from build123d import *

# Parameters (mm, degrees)
SKETCH1_W               = 120
SKETCH1_H               = 110
SKETCH1_R               = 2.15
SKETCH1_R_2             = 1.65
BOSS_EXTRUDE1_DEPTH     = 3
SKETCH2_R               = 3
SKETCH2_R_2             = 1.65
BOSS_EXTRUDE2_DEPTH     = 6.6
CHAMFER5_SIZE           = 1.6
CHAMFER5_SIZE2          = 2.771281292
CUT_EXTRUDE1_DEPTH      = 4
SKETCH4_R               = 7
SKETCH4_R_2             = 2.15
BOSS_EXTRUDE3_DEPTH     = 9
CUT_EXTRUDE2_DEPTH      = 5
CHAMFER2_SIZE           = 0.4
SKETCH6_W               = 9
SKETCH6_H               = 16
BOSS_EXTRUDE4_DEPTH     = 6
CUT_EXTRUDE3_DEPTH      = 126.87295182
CUT_EXTRUDE3_DEPTH_BACK = 126.87295182
SKETCH8_W               = 13
SKETCH8_H               = 10
SKETCH8_R               = 2.15
BOSS_EXTRUDE5_DEPTH     = 10
CUT_EXTRUDE5_DEPTH      = 5
CHAMFER9_SIZE           = 3


with BuildPart() as part:
    # Sketch1 → Boss-Extrude1 (new body)
    with BuildSketch(Plane.XY):
        Rectangle(SKETCH1_W, SKETCH1_H)
        with Locations((-39, 39)):
            Circle(SKETCH1_R, mode=Mode.SUBTRACT)
        with Locations((39, 39)):
            Circle(SKETCH1_R, mode=Mode.SUBTRACT)
        with Locations((39, -39)):
            Circle(SKETCH1_R, mode=Mode.SUBTRACT)
        with Locations((-39, -39)):
            Circle(SKETCH1_R, mode=Mode.SUBTRACT)
        with Locations((33.07, 14.94)):
            Circle(SKETCH1_R_2, mode=Mode.SUBTRACT)
        with Locations((33.07, -13)):
            Circle(SKETCH1_R_2, mode=Mode.SUBTRACT)
        with Locations((-19, -18.08)):
            Circle(SKETCH1_R_2, mode=Mode.SUBTRACT)
        with Locations((-15.1, -29.75)):
            Circle(SKETCH1_R_2, mode=Mode.SUBTRACT)
        with Locations((15.1, -46)):
            Circle(SKETCH1_R_2, mode=Mode.SUBTRACT)
    extrude(amount=BOSS_EXTRUDE1_DEPTH)

    # Sketch2 → Boss-Extrude2 (add)
    # profile 1 of 5: a face of its own
    with BuildSketch(Plane(origin=(0, 0, 0), x_dir=(-1, 0, 0), z_dir=(0, 0, -1))):
        with Locations((-33.07, -13)):
            Circle(SKETCH2_R)
        with Locations((-33.07, -13)):
            Circle(SKETCH2_R_2, mode=Mode.SUBTRACT)
    # profile 2 of 5: a face of its own
    with BuildSketch(Plane(origin=(0, 0, 0), x_dir=(-1, 0, 0), z_dir=(0, 0, -1))):
        with Locations((19, -18.08)):
            Circle(SKETCH2_R)
        with Locations((19, -18.08)):
            Circle(SKETCH2_R_2, mode=Mode.SUBTRACT)
    # profile 3 of 5: a face of its own
    with BuildSketch(Plane(origin=(0, 0, 0), x_dir=(-1, 0, 0), z_dir=(0, 0, -1))):
        with Locations((-33.07, 14.94)):
            Circle(SKETCH2_R)
        with Locations((-33.07, 14.94)):
            Circle(SKETCH2_R_2, mode=Mode.SUBTRACT)
    # profile 4 of 5: a face of its own
    with BuildSketch(Plane(origin=(0, 0, 0), x_dir=(-1, 0, 0), z_dir=(0, 0, -1))):
        with Locations((-15.1, -46)):
            Circle(SKETCH2_R)
        with Locations((-15.1, -46)):
            Circle(SKETCH2_R_2, mode=Mode.SUBTRACT)
    # profile 5 of 5: a face of its own
    with BuildSketch(Plane(origin=(0, 0, 0), x_dir=(-1, 0, 0), z_dir=(0, 0, -1))):
        with Locations((15.1, -29.75)):
            Circle(SKETCH2_R)
        with Locations((15.1, -29.75)):
            Circle(SKETCH2_R_2, mode=Mode.SUBTRACT)
    extrude(amount=-BOSS_EXTRUDE2_DEPTH)

    # Chamfer5
    chamfer5_edges = [part.edges().sort_by_distance(p)[0] for p in [
        (36.07, -13, 3),
        (-16, -18.08, 3),
        (36.07, 14.94, 3),
        (18.1, -46, 3),
        (-12.1, -29.75, 3),
    ]]
    chamfer5_side = [part.faces().sort_by_distance(p)[0] for p in [
        (-0.102522824, 0.199847736, 3),
    ]]
    chamfer(chamfer5_edges, length=CHAMFER5_SIZE, length2=CHAMFER5_SIZE2, reference=chamfer5_side[0])

    # Sketch3 → Cut-Extrude1 (cut)
    with BuildSketch(Plane(origin=(0, 0, 0), x_dir=(-1, 0, 0), z_dir=(0, 0, -1))):
        Polygon((-31.48228676, 12.19), (-29.894573519, 14.94), (-31.48228676, 17.69), (-34.65771324, 17.69), (-36.245426481, 14.94), (-34.65771324, 12.19), align=None)
        Polygon((-31.48228676, -15.75), (-29.894573519, -13), (-31.48228676, -10.25), (-34.65771324, -10.25), (-36.245426481, -13), (-34.65771324, -15.75), align=None)
        Polygon((20.58771324, -20.83), (22.175426481, -18.08), (20.58771324, -15.33), (17.41228676, -15.33), (15.824573519, -18.08), (17.41228676, -20.83), align=None)
        Polygon((16.68771324, -32.5), (18.275426481, -29.75), (16.68771324, -27), (13.51228676, -27), (11.924573519, -29.75), (13.51228676, -32.5), align=None)
        Polygon((-13.51228676, -48.75), (-11.924573519, -46), (-13.51228676, -43.25), (-16.68771324, -43.25), (-18.275426481, -46), (-16.68771324, -48.75), align=None)
    extrude(amount=-CUT_EXTRUDE1_DEPTH, mode=Mode.SUBTRACT)

    # Sketch4 → Boss-Extrude3 (add)
    # profile 1 of 4: a face of its own
    with BuildSketch(Plane(origin=(0, 0, 0), x_dir=(-1, 0, 0), z_dir=(0, 0, -1))):
        with Locations((-39, 39)):
            Circle(SKETCH4_R)
        with Locations((-39, 39)):
            Circle(SKETCH4_R_2, mode=Mode.SUBTRACT)
    # profile 2 of 4: a face of its own
    with BuildSketch(Plane(origin=(0, 0, 0), x_dir=(-1, 0, 0), z_dir=(0, 0, -1))):
        with Locations((39, 39)):
            Circle(SKETCH4_R)
        with Locations((39, 39)):
            Circle(SKETCH4_R_2, mode=Mode.SUBTRACT)
    # profile 3 of 4: a face of its own
    with BuildSketch(Plane(origin=(0, 0, 0), x_dir=(-1, 0, 0), z_dir=(0, 0, -1))):
        with Locations((39, -39)):
            Circle(SKETCH4_R)
        with Locations((39, -39)):
            Circle(SKETCH4_R_2, mode=Mode.SUBTRACT)
    # profile 4 of 4: a face of its own
    with BuildSketch(Plane(origin=(0, 0, 0), x_dir=(-1, 0, 0), z_dir=(0, 0, -1))):
        with Locations((-39, -39)):
            Circle(SKETCH4_R)
        with Locations((-39, -39)):
            Circle(SKETCH4_R_2, mode=Mode.SUBTRACT)
    extrude(amount=-BOSS_EXTRUDE3_DEPTH)

    # Sketch5 → Cut-Extrude2 (cut)
    with BuildSketch(Plane.XY.offset(9)):
        Polygon((-36.979274058, 42.5), (-41.020725942, 42.5), (-43.041451884, 39), (-41.020725942, 35.5), (-36.979274058, 35.5), (-34.958548116, 39), align=None)
        Polygon((36.979274058, 42.5), (34.958548116, 39), (36.979274058, 35.5), (41.020725942, 35.5), (43.041451884, 39), (41.020725942, 42.5), align=None)
        Polygon((36.979274058, -35.5), (34.958548116, -39), (36.979274058, -42.5), (41.020725942, -42.5), (43.041451884, -39), (41.020725942, -35.5), align=None)
        Polygon((-36.979274058, -35.5), (-41.020725942, -35.5), (-43.041451884, -39), (-41.020725942, -42.5), (-36.979274058, -42.5), (-34.958548116, -39), align=None)
    extrude(amount=-CUT_EXTRUDE2_DEPTH, mode=Mode.SUBTRACT)

    # Chamfer2
    chamfer2_edges = [part.edges().sort_by_distance(p)[0] for p in [
        (46, 39, 9),
        (-32, 39, 9),
        (-32, -39, 9),
        (46, -39, 9),
    ]]
    chamfer(chamfer2_edges, length=CHAMFER2_SIZE)

    # Sketch6 → Boss-Extrude4 (add)
    with BuildSketch(Plane.ZY.offset(60)):
        with Locations((7.5, 47)):
            Rectangle(SKETCH6_W, SKETCH6_H)
        with Locations((7.5, -47)):
            Rectangle(SKETCH6_W, SKETCH6_H)
    boss_extrude4 = extrude(amount=-BOSS_EXTRUDE4_DEPTH)

    # Mirror1: Boss-Extrude4 across plane
    add(boss_extrude4.mirror(Plane(origin=(0, 0, 0), x_dir=(0, 0, 1), z_dir=(1, 0, 0))))

    # Sketch7 → Cut-Extrude3 (cut, two sides: drawn at the far end of the back side and taken through both)
    with BuildSketch(Plane(origin=(0, 55, 0), x_dir=(1, 0, 0), z_dir=(0, 1, 0)).offset(-CUT_EXTRUDE3_DEPTH_BACK)):
        Polygon((-60, -10.5), (-57, -7.5), (-60, -4.5), align=None)
        Polygon((60, -10.5), (57, -7.5), (60, -4.5), align=None)
    extrude(amount=CUT_EXTRUDE3_DEPTH + CUT_EXTRUDE3_DEPTH_BACK, mode=Mode.SUBTRACT)

    # Sketch8 → Boss-Extrude5 (add)
    with BuildSketch(Plane(origin=(0, 55, 0), x_dir=(1, 0, 0), z_dir=(0, 1, 0))):
        with Locations((0, -8)):
            Rectangle(SKETCH8_W, SKETCH8_H)
        with Locations(Location((0, -8, 0), (0, 0, 180))):
            Circle(SKETCH8_R, mode=Mode.SUBTRACT)
    extrude(amount=-BOSS_EXTRUDE5_DEPTH)

    # Sketch9 → Cut-Extrude5 (cut)
    with BuildSketch(Plane.XZ.offset(-45)):
        Polygon((0, 12.041451884), (-3.5, 10.020725942), (-3.5, 5.979274058), (0, 3.958548116), (3.5, 5.979274058), (3.5, 10.020725942), align=None)
    extrude(amount=-CUT_EXTRUDE5_DEPTH, mode=Mode.SUBTRACT)

    # Chamfer9
    chamfer9_edges = [part.edges().sort_by_distance(p)[0] for p in [
        (-6.5, 50, 13),
        (6.5, 50, 13),
    ]]
    chamfer(chamfer9_edges, length=CHAMFER9_SIZE)


solid = part.part
Part model, mm, in its own coordinate system. A direction names the side the tool comes from. Coordinates: 2 decimals unless noted, no trailing zeros. Loops run counter-clockwise (first coordinate to the right, second up) from the corner with the lowest first, then second, coordinate; pieces in that order, holes last. Notation, with made-up numbers: M -38,53 L 3,53 A24 cw 3,66 Z; hole C -27,25.5 d9. An arc over 180 degrees is marked long. Use a Markdown table: item, result. Add a question column.
Q1. Cut at D-D (x = -25.5). Write the cut outline in (y, z).
Q2. Cut at A-A (x = 15.1). Write the cut outline in (y, z).
Q3. Cut at B-B (x = -39). Give the number of separate pieces and of enclosed holes in the cut face, and give its area (3 significant figures).
Q4. Which spindle directions (+Z, -Z, +X, -X, +Y, -Y) get a long thin tool onto all of the face, cutting with end or side? Do faces 1 (the flat face through (36, -42, 9)), 2 (the flat face through (-36, 37.2, 6.5)), 3 (the flat face through (12.71, -44.64, 1.97)), 4 (the flat face through (-1.8, 47.5, 5)). Say none if no direction does.
Q5. Mould opens along X. For faces 5 (the flat face through (12.73, -47.394, 1.972)), 6 (the flat face through (-1, 1, 0)), 7 (the flat face through (30.7, -14.394, 1.972)) say: +X half, -X half, draft (parallel to the pull), parting line (faces both ways), or undercut.
Q6. Cut at C-C (y = -2.5). Write the cut outline in (x, z), and give its area (3 significant figures).
Q7. Probe L1, parallel to Y at x = -39, z = 3.3; L2, parallel to Y at x = 54.5, z = 5.5; L3, parallel to X at y = -46, z = 1.75. List the from-to ranges inside material, lowest first.
Q8. Pin check, flat tips, straight feed: P1, Ø10, axis at x = 10, y = 22.5, coming from the +Z side; P2, Ø5, axis at y = -35.5, z = 5, coming from the -X side; P3, Ø6.5, axis at x = 33.5, y = -12, coming from the +Z side; P4, Ø3.5, axis at x = -39, y = 39, coming from the -Z side. Stop position of each tip, or through.
Worked out:
| question | item | result |
|---|---|---|
| 1 | outline | M -55,0 L 55,0 L 55,3 L -55,3 Z |
| 2 | outline | M -55,0 L -48.75,0 L -48.75,4 L -47.65,4 L -47.65,6.6 L -49,6.6 L -49,5.77 L -50.6,3 L -55,3 Z; M -44.35,4 L -43.25,4 L -43.25,0 L 55,0 L 55,3 L -41.4,3 L -43,5.77 L -43,6.6 L -44.35,6.6 Z |
| 3 | separate pieces | 3 |
| 3 | enclosed holes | 0 |
| 3 | area | 393 mm2 |
| 4 | face 1 | +Z, +Y, -Y |
| 4 | face 2 | +Z |
| 4 | face 3 | -Z |
| 4 | face 4 | -Y |
| 5 | face 5 | undercut |
| 5 | face 6 | draft |
| 5 | face 7 | undercut |
| 6 | outline | M -60,0 L 60,0 L 60,3 L -60,3 Z |
| 6 | area | 360 mm2 |
| 7 | L1 | y = -46 to -41.15, -36.85 to -32, 32 to 36.85, 41.15 to 46 |
| 7 | L2 | y = -55 to -39, 39 to 55 |
| 7 | L3 | x = -60 to 11.92, 18.28 to 60 |
| 8 | P1 | stops at z = 3 |
| 8 | P2 | stops at x = -60 |
| 8 | P3 | stops at z = 6.6 |
| 8 | P4 | passes through |
